Can you work these out from the model? Positions are in its coordinate system, mm. Face numbers are marked on the shaded views. A direction names the side the tool comes from. Give positions to 0.01 mm unless a question says otherwise; leave off trailing zeros. Order: outer loops, then holes, each group sorted by start corner. A loop starts at its lowest first (then second) coordinate and runs counter-clockwise, first axis right, second up. Notation, with made-up numbers: (-8, 89) - (10, 89) arc R33 cw to (10, 121) - close; hole circle Ø6 at (22, -28.5). An arc over 180 degrees is marked (long way). Answer as a JSON object with one key per item and string values.
```python
from build123d import *

# Parameters (mm, degrees)
SKETCH1_W            = 15.875
SKETCH1_H            = 15.875
BOSS_EXTRUDE1_DEPTH  = 11.938
SKETCH2_W            = 10.922
SKETCH2_H            = 6.35
BOSS_EXTRUDE2_DEPTH  = 2.413
SKETCH3_W            = 5.334
SKETCH3_H            = 8.128
BOSS_EXTRUDE3_DEPTH  = 1.524
SKETCH4_W            = 6.096
SKETCH4_H            = 5.334
BOSS_EXTRUDE4_DEPTH  = 2.286
SKETCH5_R            = 1.7145
BOSS_EXTRUDE5_DEPTH  = 1.778
SKETCH6_R            = 1.397
BOSS_EXTRUDE6_DEPTH  = 4.318
SKETCH7_W            = 9.779
SKETCH7_H            = 11.43
BOSS_EXTRUDE7_DEPTH  = 3.175
SKETCH8_W            = 11.43
SKETCH8_H            = 9.779
BOSS_EXTRUDE8_DEPTH  = 3.175
SKETCH9_R            = 2.413
SKETCH9_R_2          = 1.8415
CUT_EXTRUDE1_DEPTH   = 0.508
SKETCH10_R           = 2.413
SKETCH10_R_2         = 1.8415
CUT_EXTRUDE2_DEPTH   = 0.508
SKETCH12_W           = 0.508
SKETCH12_H           = 4.445
EXTRUDE_THIN1_DEPTH  = 1.016
SKETCH13_W           = 0.508
SKETCH13_H           = 4.445
EXTRUDE_THIN2_DEPTH  = 1.016
FILLET1_R            = 0.508
BOSS_EXTRUDE9_DEPTH  = 0.254
BOSS_EXTRUDE10_DEPTH = 0.254
SKETCH16_W           = 0.254
SKETCH16_H           = 0.508
BOSS_EXTRUDE11_DEPTH = 2.54
CHAMFER1_SIZE        = 0.254


with BuildPart() as part:
    # Sketch1 → Boss-Extrude1 (new body)
    with BuildSketch(Plane.XY):
        with Locations((7.9375, 7.9375)):
            Rectangle(SKETCH1_W, SKETCH1_H)
    extrude(amount=BOSS_EXTRUDE1_DEPTH)

    # Sketch2 → Boss-Extrude2 (add)
    with BuildSketch(Plane(origin=(0, 0, 0), x_dir=(-1, 0, 0), z_dir=(0, 0, -1))):
        with Locations((-7.9375, 19.05)):
            Rectangle(SKETCH2_W, SKETCH2_H)
    extrude(amount=-BOSS_EXTRUDE2_DEPTH)

    # Sketch3 → Boss-Extrude3 (add)
    with BuildSketch(Plane(origin=(15.875, 0, 0), x_dir=(0, 0, -1), z_dir=(1, 0, 0))):
        with Locations((-2.667, 7.9375)):
            Rectangle(SKETCH3_W, SKETCH3_H)
    extrude(amount=BOSS_EXTRUDE3_DEPTH)

    # Sketch4 → Boss-Extrude4 (add)
    with BuildSketch(Plane.XY.offset(2.413)):
        with Locations((7.9375, 18.542)):
            Rectangle(SKETCH4_W, SKETCH4_H)
    extrude(amount=BOSS_EXTRUDE4_DEPTH)

    # Sketch5 → Boss-Extrude5 (add)
    with BuildSketch(Plane.XY.offset(4.699)):
        with Locations(Location((7.9375, 18.542, 0), (0, 0, 180))):
            Circle(SKETCH5_R)
    extrude(amount=BOSS_EXTRUDE5_DEPTH)

    # Sketch6 → Boss-Extrude6 (add)
    with BuildSketch(Plane(origin=(0, 15.875, 0), x_dir=(1, 0, 0), z_dir=(0, 1, 0))):
        with Locations(Location((7.9375, -8.090189982, 0), (0, 0, 90))):
            Circle(SKETCH6_R)
    extrude(amount=BOSS_EXTRUDE6_DEPTH)



with BuildPart() as body_2:
    # Sketch7 → Boss-Extrude7 (new body)
    with BuildSketch(Plane.XZ):
        with Locations((7.9375, 6.223)):
            Rectangle(SKETCH7_W, SKETCH7_H)
    extrude(amount=BOSS_EXTRUDE7_DEPTH)

    # Sketch10 → Cut-Extrude2 (cut)
    # profile 1 of 5: a face of its own
    with BuildSketch(Plane.XZ.offset(3.175)):
        with Locations(Location((7.9375, 6.858, 0), (0, 0, 270))):
            Circle(SKETCH10_R)
        with Locations(Location((7.9375, 6.858, 0), (0, 0, 270))):
            Circle(SKETCH10_R_2, mode=Mode.SUBTRACT)
    # profile 2 of 5: a face of its own
    with BuildSketch(Plane.XZ.offset(3.175)):
        with BuildLine():
            Line((3.429447205, 7.62), (4.98628669, 7.62))
            ThreePointArc((4.98628669, 7.62), (5.782238531, 9.013261469), (7.1755, 9.80921331))
            Line((7.1755, 9.80921331), (7.1755, 11.366052795))
            ThreePointArc((7.1755, 11.366052795), (4.704607796, 10.090892204), (3.429447205, 7.62))
        make_face()
    # profile 3 of 5: a face of its own
    with BuildSketch(Plane.XZ.offset(3.175)):
        with BuildLine():
            Line((3.429447205, 6.096), (4.98628669, 6.096))
            ThreePointArc((4.98628669, 6.096), (5.782238531, 4.702738531), (7.1755, 3.90678669))
            Line((7.1755, 3.90678669), (7.1755, 2.349947205))
            ThreePointArc((7.1755, 2.349947205), (4.704607796, 3.625107796), (3.429447205, 6.096))
        make_face()
    # profile 4 of 5: a face of its own
    with BuildSketch(Plane.XZ.offset(3.175)):
        with BuildLine():
            Line((8.6995, 11.366052795), (8.6995, 9.80921331))
            ThreePointArc((8.6995, 9.80921331), (10.092761469, 9.013261469), (10.88871331, 7.62))
            Line((10.88871331, 7.62), (12.445552795, 7.62))
            ThreePointArc((12.445552795, 7.62), (11.170392204, 10.090892204), (8.6995, 11.366052795))
        make_face()
    # profile 5 of 5: a face of its own
    with BuildSketch(Plane.XZ.offset(3.175)):
        with BuildLine():
            Line((12.445552795, 6.096), (10.88871331, 6.096))
            ThreePointArc((10.88871331, 6.096), (10.092761469, 4.702738531), (8.6995, 3.90678669))
            Line((8.6995, 3.90678669), (8.6995, 2.349947205))
            ThreePointArc((8.6995, 2.349947205), (11.170392204, 3.625107796), (12.445552795, 6.096))
        make_face()
    extrude(amount=-CUT_EXTRUDE2_DEPTH, mode=Mode.SUBTRACT)


with BuildPart() as body_3:
    # Sketch8 → Boss-Extrude8 (new body)
    with BuildSketch(Plane.ZY):
        with Locations((6.223, 7.9375)):
            Rectangle(SKETCH8_W, SKETCH8_H)
    extrude(amount=BOSS_EXTRUDE8_DEPTH)

    # Sketch9 → Cut-Extrude1 (cut)
    # profile 1 of 5: a face of its own
    with BuildSketch(Plane.ZY.offset(3.175)):
        with Locations((6.858, 7.9375)):
            Circle(SKETCH9_R)
        with Locations((6.858, 7.9375)):
            Circle(SKETCH9_R_2, mode=Mode.SUBTRACT)
    # profile 2 of 5: a face of its own
    with BuildSketch(Plane.ZY.offset(3.175)):
        with BuildLine():
            Line((7.62, 12.445552795), (7.62, 10.88871331))
            ThreePointArc((7.62, 10.88871331), (9.013261469, 10.092761469), (9.80921331, 8.6995))
            Line((9.80921331, 8.6995), (11.366052795, 8.6995))
            ThreePointArc((11.366052795, 8.6995), (10.090892204, 11.170392204), (7.62, 12.445552795))
        make_face()
    # profile 3 of 5: a face of its own
    with BuildSketch(Plane.ZY.offset(3.175)):
        with BuildLine():
            Line((6.096, 12.445552795), (6.096, 10.88871331))
            ThreePointArc((6.096, 10.88871331), (4.702738531, 10.092761469), (3.90678669, 8.6995))
            Line((3.90678669, 8.6995), (2.349947205, 8.6995))
            ThreePointArc((2.349947205, 8.6995), (3.625107796, 11.170392204), (6.096, 12.445552795))
        make_face()
    # profile 4 of 5: a face of its own
    with BuildSketch(Plane.ZY.offset(3.175)):
        with BuildLine():
            Line((11.366052795, 7.1755), (9.80921331, 7.1755))
            ThreePointArc((9.80921331, 7.1755), (9.013261469, 5.782238531), (7.62, 4.98628669))
            Line((7.62, 4.98628669), (7.62, 3.429447205))
            ThreePointArc((7.62, 3.429447205), (10.090892204, 4.704607796), (11.366052795, 7.1755))
        make_face()
    # profile 5 of 5: a face of its own
    with BuildSketch(Plane.ZY.offset(3.175)):
        with BuildLine():
            Line((6.096, 3.429447205), (6.096, 4.98628669))
            ThreePointArc((6.096, 4.98628669), (4.702738531, 5.782238531), (3.90678669, 7.1755))
            Line((3.90678669, 7.1755), (2.349947205, 7.1755))
            ThreePointArc((2.349947205, 7.1755), (3.625107796, 4.704607796), (6.096, 3.429447205))
        make_face()
    extrude(amount=-CUT_EXTRUDE1_DEPTH, mode=Mode.SUBTRACT)


with BuildPart() as part_1:
    add(part.part)

    add(body_3.part)  # Revolve1 merges body 3

    add(body_2.part)  # Revolve1 merges body 2
    # Sketch11 → Revolve1 (revolve)
    with BuildSketch(Plane(origin=(7.9375, 7.9375, 0), x_dir=(-0.7071067811865475, 0.7071067811865477, 0), z_dir=(-0.7071067811865477, -0.7071067811865475, 0)), mode=Mode.PRIVATE) as revolve1_sk:
        with BuildLine():
            Line((0, -11.938), (0, -30.226))
            add(Edge.make_bspline(
                [(9.906, -25.781), (9.751729045, -27.856462125), (6.04050774, -30.161976774), (0, -30.226)],
                knots=[0, 0, 0, 0, 1, 1, 1, 1], degree=3))
            Line((9.906, -25.781), (5.588, -24.511))
            Line((5.588, -24.511), (5.588, -19.685))
            add(Edge.make_bspline(
                [(5.588, -19.685), (10.703599442, -19.17170065), (12.337124929, -16.678247384), (13.335, -11.43)],
                knots=[0, 0, 0, 0, 1, 1, 1, 1], degree=3))
            Line((13.335, -11.43), (12.81776957, -11.43))
            add(Edge.make_bspline(
                [(5.08, -19.225421832), (5.399913167, -19.193321739), (6.061720289, -19.129363969), (7.20278515, -18.93540179), (8.438114269, -18.57623304), (9.614134976, -17.958168192), (10.555522363, -17.145380616), (11.317238514, -16.106567706), (11.935580098, -14.811198195), (12.353250651, -13.497363461), (12.632984775, -12.344667479), (12.761465886, -11.721646833), (12.81776957, -11.43)],
                knots=[-0.02979657, -0.02979657, -0.02979657, -0.02979657, 0.034565716, 0.098928001, 0.227652573, 0.356377144, 0.485101715, 0.613826286, 0.742550858, 0.871275429, 0.935637714, 0.993693442, 0.993693442, 0.993693442, 0.993693442], degree=3))
            Line((5.08, -19.225421832), (3.1115, -15.178653632))
            Line((3.1115, -15.178653632), (3.1115, -11.938))
            Line((3.1115, -11.938), (0, -11.938))
        make_face()
    revolve(revolve1_sk.sketch.rotate(Axis((7.9375, 7.9375, -0.5969), (0, 0, 1)), 45), axis=Axis((7.9375, 7.9375, -0.5969), (0, 0, 1)))

    # Sketch12 → Extrude-Thin1 (add)
    with BuildSketch(Plane.XZ):
        with Locations((0.254, -2.2225)):
            Rectangle(SKETCH12_W, SKETCH12_H)
        with Locations((15.621, -2.2225)):
            Rectangle(SKETCH12_W, SKETCH12_H)
    extrude(amount=-EXTRUDE_THIN1_DEPTH)

    # Sketch13 → Extrude-Thin2 (add)
    with BuildSketch(Plane(origin=(0, 15.875, 0), x_dir=(1, 0, 0), z_dir=(0, 1, 0))):
        with Locations((0.254, 2.2225)):
            Rectangle(SKETCH13_W, SKETCH13_H)
        with Locations((15.621, 2.2225)):
            Rectangle(SKETCH13_W, SKETCH13_H)
    extrude(amount=-EXTRUDE_THIN2_DEPTH)

    # Fillet1
    fillet1_edges = [part_1.edges().sort_by_distance(p)[0] for p in [
        (0.254, 1.016, -4.445),
        (0.254, 15.875, -4.445),
        (0.254, 14.859, -4.445),
        (15.621, 15.875, -4.445),
        (15.621, 14.859, -4.445),
        (15.621, 1.016, -4.445),
        (15.621, 0, -4.445),
        (0.254, 0, -4.445),
    ]]
    fillet(fillet1_edges, radius=FILLET1_R - 0.0001)  # a hair under: the kernel refuses the full size

    # Sketch14 → Boss-Extrude9 (add, symmetric)
    with BuildSketch(Plane(origin=(0, -1.5875, 0), x_dir=(-1, 0, 0), z_dir=(0, -1, 0))):
        Polygon((-10.0965, -0.508), (-10.0965, 3.697342898), (-10.4775, 4.298407671), (-10.8585, 3.697342898), (-10.8585, -0.508), align=None)
        Polygon((-7.5565, -0.508), (-7.5565, 3.697342898), (-7.9375, 4.298407671), (-8.3185, 3.697342898), (-8.3185, -0.508), align=None)
        Polygon((-5.0165, -0.508), (-5.0165, 3.697342898), (-5.3975, 4.298407671), (-5.7785, 3.697342898), (-5.7785, -0.508), align=None)
    extrude(amount=BOSS_EXTRUDE9_DEPTH, both=True)

    # Sketch15 → Boss-Extrude10 (add, symmetric)
    with BuildSketch(Plane.ZY.offset(1.5875)):
        Polygon((0.508, 8.3185), (-3.697342898, 8.3185), (-4.298407671, 7.9375), (-3.697342898, 7.5565), (0.508, 7.5565), align=None)
        Polygon((0.508, 5.7785), (-3.697342898, 5.7785), (-4.298407671, 5.3975), (-3.697342898, 5.0165), (0.508, 5.0165), align=None)
        Polygon((0.508, 10.8585), (-3.697342898, 10.8585), (-4.298407671, 10.4775), (-3.697342898, 10.0965), (0.508, 10.0965), align=None)
    extrude(amount=BOSS_EXTRUDE10_DEPTH, both=True)

    # Sketch16 → Boss-Extrude11 (add)
    with BuildSketch(Plane(origin=(0, 0, 0), x_dir=(-1, 0, 0), z_dir=(0, 0, -1))):
        with Locations((-11.2395, 20.447)):
            Rectangle(SKETCH16_W, SKETCH16_H)
        with Locations((-4.3815, 20.447)):
            Rectangle(SKETCH16_W, SKETCH16_H)
        with Locations((-4.3815, 16.129)):
            Rectangle(SKETCH16_W, SKETCH16_H)
        with Locations((-11.2395, 16.129)):
            Rectangle(SKETCH16_W, SKETCH16_H)
    extrude(amount=BOSS_EXTRUDE11_DEPTH)

    # Chamfer1
    chamfer1_edges = [part_1.edges().sort_by_distance(p)[0] for p in [
        (11.2395, 15.875, -2.54),
        (11.2395, 16.383, -2.54),
        (4.3815, 15.875, -2.54),
        (4.3815, 16.383, -2.54),
        (4.3815, 20.193, -2.54),
        (4.3815, 20.701, -2.54),
        (11.2395, 20.193, -2.54),
        (11.2395, 20.701, -2.54),
    ]]
    chamfer(chamfer1_edges, length=CHAMFER1_SIZE - 0.0001)  # a hair under: the kernel refuses the full size


solid = part_1.part
```
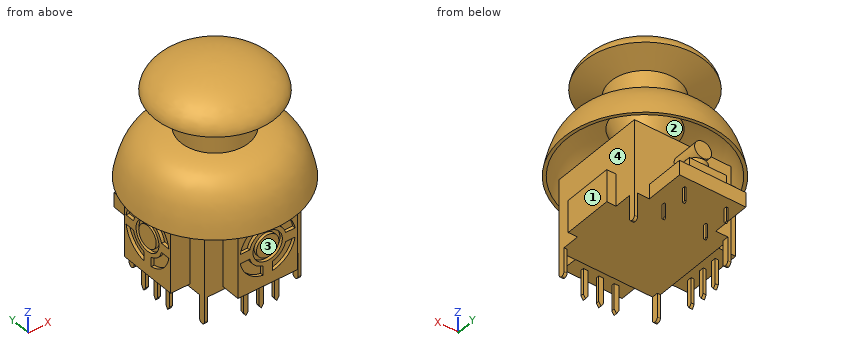
Q1. I need wall thicknesses on L1, parallel to X at y = 10.5, z = 15; L2, parallel to Z at x = 11, y = -0.5; L3, parallel to Z at x = 4, y = 13.25. Which ranges of each line are inside material? Lowest first, please.
Recorded:
{"L1": "x = -4.16 to -3.6, 6.17 to 9.7, 19.48 to 20.04", "L2": "z = 0.51 to 11.94, 18.28 to 18.84, 25.51 to 27.52", "L3": "z = 0 to 11.94, 19.03 to 19.55, 24.81 to 29.01"}
Q2. I'm going to push flat-ended pins straight in: pin 1 Ø12 at (x, y) = (3.5, 9.5) entering from -Z; pin 2 Ø2.5 at (x, y) = (8, 18.5) entering from +Z; pin 3 Ø1.1 at (y, z) = (5, 10) entering from -X (3 decimals); pin 4 Ø12 at (x, y) = (2.5, 5.5) entering from +Z. Where does each tip first touch, or does it pass through?
Recorded:
{"pin 1": "stops at z = -4.3", "pin 2": "stops at z = 27.14", "pin 3": "stops at x = -3.175", "pin 4": "stops at z = 30.23"}
Q3. We'd pull the mould along Z, two halves only. Please class the marked faces 3 and 4: released by +Z, released by -Z, zero draft, split by the parting line, or undercut.
Recorded:
{"face 3": "zero draft", "face 4": "undercut"}
Q4. If we section it at A-A, the plane y = 1.5: Count the separate pieces of the cut face and the enclosed holes in it, then the cut area to 3 significant figures.
Recorded:
{"separate pieces": "3", "enclosed holes": "0", "area": "255 mm^2"}
Q5. If we section it at B-B, the plane z = 22: Please give me the cut outline in (x, y), then the cut area to 3 significant figures.
Recorded:
{"outline": "circle Ø11.18 at (7.94, 7.94)", "area": "98.1 mm^2"}
Q6. Which directions (+Z, -Z, +X, -X, +Y, -Y) give clear straight access to the entire face, cutting with the end or side of a thin tool? Please do the marked faces 1 and 2.
Recorded:
{"face 1": "-Z, +X, +Y, -Y", "face 2": "none"}
